Could you check a few things on this drawing? It's one solid part, dimensions in mm from its lowest x, y, z. Round coordinates to 2 decimals unless told otherwise and drop trailing zeros. Loops run counter-clockwise (first coordinate to the right, second up) from the corner with the lowest first, then second, coordinate; pieces in that order, holes last. Notation, with made-up numbers: M 29,15 L 56,15 A3 ccw 56,19 Z; hole C 54,5 d8. An arc over 180 degrees is marked long. Answer as CSV lines item,"result".
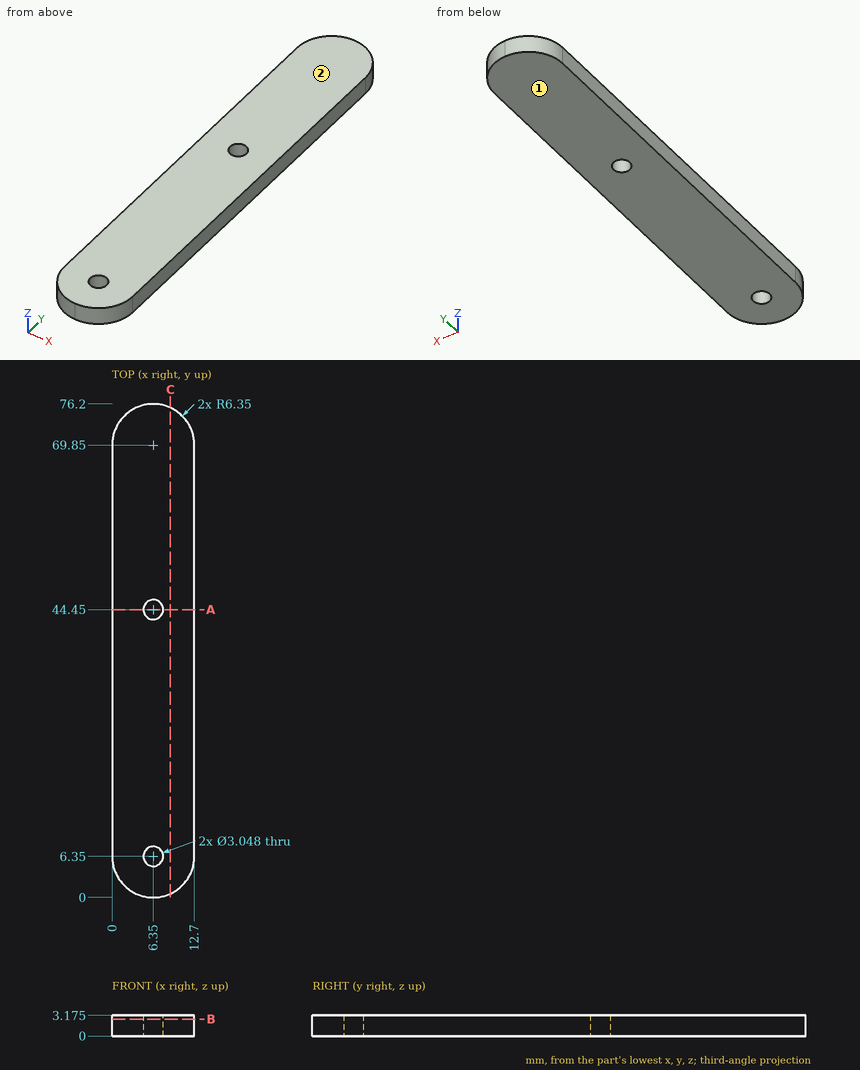
Item 1: Will these pins go through, and if not, where does the flat tip stop? pin 1 (1 mm diameter, centred on x = 1.5, z = 0.5, fed in from +Y); pin 2 (6 mm diameter, centred on x = 2, y = 18, fed in from -Z).
Output:
pin 1,"stops at y = 74.48"
pin 2,"stops at z = 0"
Item 2: If we section it at C-C on x = 9: Write out the boundary of the cut face in (y, z) (3 decimals).
Output:
outline,"M 0.579,0 L 75.621,0 L 75.621,3.175 L 0.579,3.175 Z"
Item 3: If we section it at A-A on y = 44.45: Write out the boundary of the cut face in (x, z) (3 decimals).
Output:
outline,"M 0,0 L 4.826,0 L 4.826,3.175 L 0,3.175 Z; M 7.874,0 L 12.7,0 L 12.7,3.175 L 7.874,3.175 Z"
Item 4: We'd pull the mould along Z, two halves only. Please class the marked faces 1 and 2: released by +Z, released by -Z, zero draft, split by the parting line, or undercut.
Output:
face 1,"released by -Z"
face 2,"released by +Z"
Item 5: If we section it at B-B on z = 2.6: Write out the boundary of the cut face in (x, y), then the cut area to 3 significant figures.
Output:
outline,"M 0,6.35 A6.35 ccw 12.7,6.35 L 12.7,69.85 A6.35 ccw 0,69.85 Z; hole C 6.35,6.35 d3.05; hole C 6.35,44.45 d3.05"
area,"919 mm2"
Item 6: If I drill on line 1 along Y through (x, z) = (7.5, 2.9) (3 decimals); line 2 along Y through (x, z) = (7, 2.4); line 3 along X through (y, z) = (6, 1.7), over which ranges is the centre line in solid material (lowest first)? Write a range as from..to.
Output:
line 1,"y = 0.105..5.35, 7.35..43.45, 45.45..76.095"
line 2,"y = 0.03..4.97, 7.73..43.07, 45.83..76.17"
line 3,"x = 0.01..4.87, 7.83..12.69"
